Could you check a few things on this model? Use its own coordinates, in mm. A direction names the side the tool comes from. Coordinates: 2 decimals unless noted, no trailing zeros. Loops run counter-clockwise (first coordinate to the right, second up) from the corner with the lowest first, then second, coordinate; pieces in that order, holes last. Notation, with made-up numbers: (1, 7) - (47, 7) arc R12 cw to (47, 22) - close; hole circle Ø9 at (49.5, 26.5). An arc over 180 degrees is marked (long way). One line per item, written item: value. Start each with the question number.
(1) On a 3-axis mill with a long thin cutter (end or side, diameter ignored), from which of +Z, -Z, +X, -X, +Y, -Y can I reach the whole of each face in a straight line? I mean faces 1 (the face through (5, 0.4, 0)), 2 (the face through (-9.09, 4.28, 0.04)), 3 (the face through (-9, -6, 0)), 4 (the face through (-19.699, 7.715, 0.049)). Say none if no direction works.
(2) If we section it at A-A on x = 16: Write out the boundary of the cut face in (y, z), then the cut area to 3 significant figures.
(3) I'm going to push a flat-ended pin straight in: P1, Ø1.3, axis at x = -6.5, z = -1, coming from the -Y side. Where does the tip first touch, or does it pass through?
(4) If I drill on line 1 along Y through (x, z) = (0, 1); line 2 along X through (y, z) = (-4.35, 0); line 3 along X through (y, z) = (2, 1), over which ranges is the centre line in solid material (lowest first)? Write a range as from..to.
(5) If we section it at C-C on z = -3: Count the separate pieces of the cut face and the enclosed holes in it, then the cut area to 3 significant figures.
(6) If we section it at D-D on x = -6: Write out the boundary of the cut face in (y, z).
(7) If we mould it in two halves opening along X, with no side actions, what happens to faces 5 (the face through (5, -0.4, 0)), 6 (the face through (19.715, 7.699, 0.049)), 7 (the face through (1, 8, 0)), 8 (the face through (-7, 4, -1.6))? For each: pulls with the +X half, pulls with the -X half, needs draft (parallel to the pull), parting line crosses it, or undercut.
(8) If we section it at B-B on y = -8: Write out the boundary of the cut face in (x, z), then the cut area to 3 significant figures.
```python
from build123d import *

# Parameters (mm, degrees)
BOSS_EXTRUDE1_DEPTH      = 3.5
BOSS_EXTRUDE1_DEPTH_BACK = 3.5
SKETCH1_R                = 1.6
CUT_EXTRUDE1_REACH       = 30.5
SKETCH3_R                = 1.6
SKETCH3_3_R              = 2.2
SKETCH3_3_R_2            = 1.6
CUT_EXTRUDE2_DEPTH       = 6
CUT_EXTRUDE3_REACH       = 30.5
FILLET1_R                = 1
FILLET2_R                = 0.4


with BuildPart() as part:
    # Sketch1 → Boss-Extrude1 (new, two sides: drawn at the far end of the back side and taken through both)
    with BuildSketch(Plane.XY.offset(-BOSS_EXTRUDE1_DEPTH_BACK)):
        with BuildLine():
            Line((-20, 8), (-18.64966284, 8))
            Line((-18.64966284, 8), (-10, -0.5))
            Line((-10, -0.5), (-3.979949748, -0.4))
            ThreePointArc((-3.979949748, -0.4), (0, -4), (3.979949748, -0.4))
            Line((3.979949748, -0.4), (6, -0.4))
            Line((6, -0.4), (6, 0.4))
            Line((6, 0.4), (3.979949748, 0.4))
            ThreePointArc((3.979949748, 0.4), (0, 4), (-3.979949748, 0.4))
            Line((-3.979949748, 0.4), (-10, 0.5))
            Line((-10, 0.5), (-16.848441102, 8))
            Line((-16.848441102, 8), (20, 8))
            Line((20, 8), (20, -12))
            Line((20, -12), (-20, -12))
            Line((-20, -12), (-20, 8))
        make_face()
        with Locations((-16, 0)):
            Circle(SKETCH1_R, mode=Mode.SUBTRACT)
        with Locations(Location((16, 0, 0), (0, 0, 180))):
            Circle(SKETCH1_R, mode=Mode.SUBTRACT)
        with Locations((0, -8)):
            Circle(SKETCH1_R, mode=Mode.SUBTRACT)
    extrude(amount=BOSS_EXTRUDE1_DEPTH + BOSS_EXTRUDE1_DEPTH_BACK)

    # Cut-Extrude1: up to this plane
    cut_extrude1_end = Plane(origin=(-10, -0.5, -3.5), z_dir=(-0.016608865731892127, 0.9998620632762801, 0))
    # Sketch3 → Cut-Extrude1 (cut, up to the surface)
    with BuildSketch(Plane.XZ.offset(12), mode=Mode.PRIVATE) as cut_extrude1_sk1:
        with Locations(Location((-6.989974874, 0, 0), (0, 0, 270))):
            Circle(SKETCH3_R)
    cut_extrude1_tool1 = split(extrude(cut_extrude1_sk1.sketch, amount=-CUT_EXTRUDE1_REACH, mode=Mode.PRIVATE), bisect_by=cut_extrude1_end, keep=Keep.BOTH, mode=Mode.PRIVATE)
    add(cut_extrude1_tool1.solids().sort_by_distance((-6.989975, -12, 0))[0], mode=Mode.SUBTRACT)

    # Sketch3<3> → Cut-Extrude2 (cut)
    with BuildSketch(Plane.XZ.offset(12)):
        with Locations(Location((-6.989974874, 0, 0), (0, 0, 270))):
            Circle(SKETCH3_3_R)
        with Locations(Location((-6.989974874, 0, 0), (0, 0, 270))):
            Circle(SKETCH3_3_R_2, mode=Mode.SUBTRACT)
    extrude(amount=-CUT_EXTRUDE2_DEPTH, mode=Mode.SUBTRACT)

    # Cut-Extrude3: up to this plane
    cut_extrude3_end = Plane(origin=(-10, 0.5, -3.5), z_dir=(-0.016608865731892127, -0.9998620632762801, 0))
    # Sketch4 → Cut-Extrude3 (cut, up to the surface)
    with BuildSketch(Plane(origin=(0, 8, 0), x_dir=(1, 0, 0), z_dir=(0, 1, 0)), mode=Mode.PRIVATE) as cut_extrude3_sk1:
        with BuildLine():
            Line((-7.489974874, 1.6), (-6.489974874, 1.6))
            ThreePointArc((-6.489974874, 1.6), (-4.889974874, 0), (-6.489974874, -1.6))
            Line((-6.489974874, -1.6), (-7.489974874, -1.6))
            ThreePointArc((-7.489974874, -1.6), (-9.089974874, 0), (-7.489974874, 1.6))
        make_face()
    cut_extrude3_tool1 = split(extrude(cut_extrude3_sk1.sketch, amount=-CUT_EXTRUDE3_REACH, mode=Mode.PRIVATE), bisect_by=cut_extrude3_end, keep=Keep.BOTH, mode=Mode.PRIVATE)
    add(cut_extrude3_tool1.solids().sort_by_distance((-6.989975, 8, 0))[0], mode=Mode.SUBTRACT)

    # Fillet1
    fillet1_edges = [part.edges().sort_by_distance(p)[0] for p in [
        (20, 8, 0),
        (20, -12, 0),
        (-20, -12, 0),
        (-20, 8, 0),
    ]]
    fillet(fillet1_edges, radius=FILLET1_R)

    # Fillet2
    fillet2_edges = [part.edges().sort_by_distance(p)[0] for p in [
        (6, -0.4, 0),
        (6, 0.4, 0),
    ]]
    fillet(fillet2_edges, radius=FILLET2_R - 0.0001)  # a hair under: the kernel refuses the full size


solid = part.part
```
Values:
1. face 1: +Z, -Z
1. face 2: +Y
1. face 3: -Y
1. face 4: +Z, -Z, -X, +Y
2. outline: (-12, -3.5) - (-1.6, -3.5) - (-1.6, 3.5) - (-12, 3.5) - close; (1.6, -3.5) - (8, -3.5) - (8, 3.5) - (1.6, 3.5) - close
2. area: 118 mm2
3. P1: stops at y = -6
4. line 1: y = -12..-9.6, -6.4..-4, 4..8
4. line 2: x = -20..-8.59, -5.39..20
4. line 3: x = -20..-12.54, -11.37..-8.74, -5.24..-3.46, 3.46..20
5. separate pieces: 1
5. enclosed holes: 3
5. area: 707 mm2
6. outline: (-12, -3.5) - (-0.43, -3.5) - (-0.43, -1.26) - (-6, -1.26) - (-6, -1.96) - (-12, -1.96) - close; (-12, 1.96) - (-6, 1.96) - (-6, 1.26) - (-0.43, 1.26) - (-0.43, 3.5) - (-12, 3.5) - close; (0.43, -3.5) - (8, -3.5) - (8, -1.52) - (0.43, -1.52) - close; (0.43, 1.52) - (8, 1.52) - (8, 3.5) - (0.43, 3.5) - close
7. face 5: undercut
7. face 6: pulls with the +X half
7. face 7: needs draft
7. face 8: undercut
8. outline: (-20, -3.5) - (-1.6, -3.5) - (-1.6, 3.5) - (-20, 3.5) - close; (1.6, -3.5) - (20, -3.5) - (20, 3.5) - (1.6, 3.5) - close; hole circle Ø4.4 at (-6.99, 0)
8. area: 242 mm2
